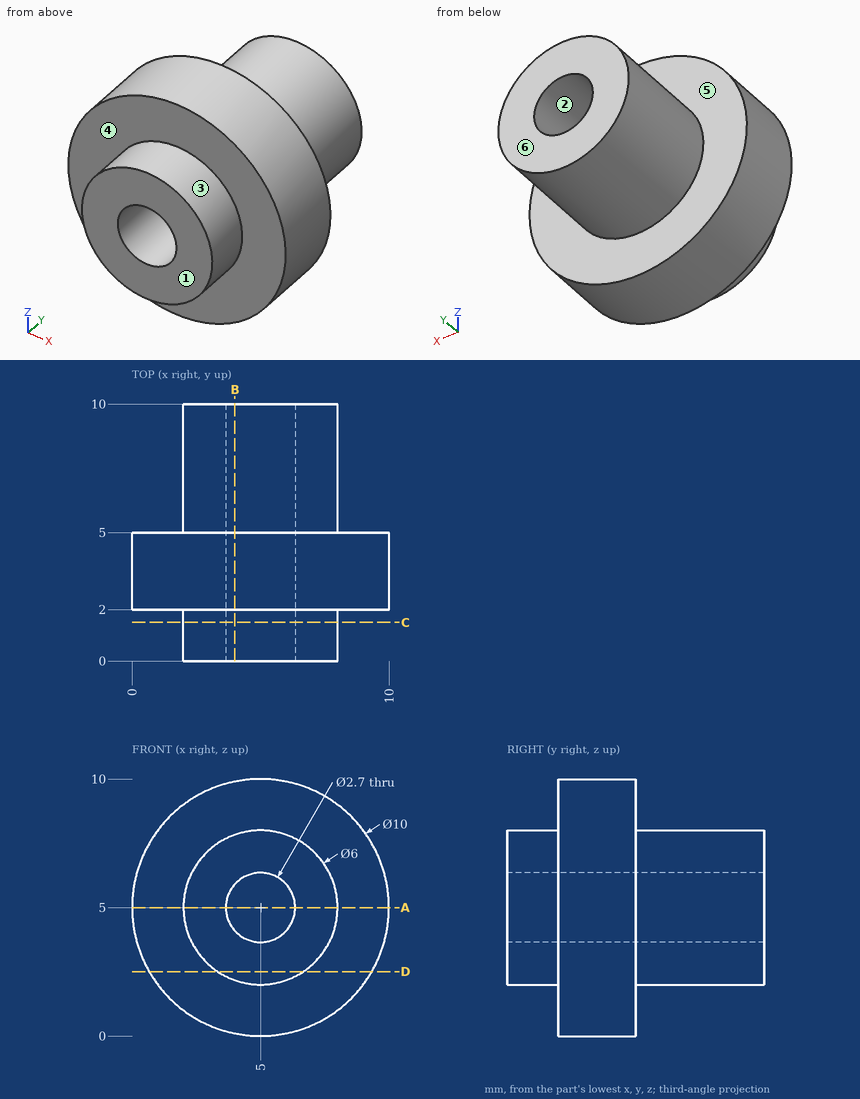
Check sheet for the drawn part. Datum: minimum x, y, z corner. Units: mm. A direction names the side the tool comes from. Round coordinates to 2 decimals unless told otherwise and drop trailing zeros. Write each loop counter-clockwise with the first axis right and the second up, starting at its lowest first coordinate (ties: lowest second). Pieces come first, ordered by that corner, then holes. Notation, with made-up numbers: (66, 14.25) -> (110, 14.25) arc R12 ccw to (110, 20.25) -> close; hole circle Ø6 at (17, 66). An arc over 180 degrees is marked (long way). Write each question's results on one line, items separated by ' | '.
Q1. Access from +Z, -Z, +X, -X, +Y, -Y to the whole of each face (thin tool, end or side, straight path). Record for the marked faces 4, 5 and 6.
Derived:
face 4: -Y | face 5: +Y | face 6: +Z, -Z, +X, -X, +Y
Q2. Sectioned sample at B-B, the plane x = 4. Record the boundary of the cut face in (y, z).
Derived:
outline: (0, 2.17) -> (2, 2.17) -> (2, 0.1) -> (5, 0.1) -> (5, 2.17) -> (10, 2.17) -> (10, 4.09) -> (0, 4.09) -> close; (0, 5.91) -> (10, 5.91) -> (10, 7.83) -> (5, 7.83) -> (5, 9.9) -> (2, 9.9) -> (2, 7.83) -> (0, 7.83) -> close
Q3. Sectioned sample at D-D, the plane z = 2.5. Record the boundary of the cut face in (x, y).
Derived:
outline: (0.67, 2) -> (3.34, 2) -> (3.34, 0) -> (6.66, 0) -> (6.66, 2) -> (9.33, 2) -> (9.33, 5) -> (6.66, 5) -> (6.66, 10) -> (3.34, 10) -> (3.34, 5) -> (0.67, 5) -> close
Q4. Draft check along X on the marked faces 1, 2 and 3. Enter one of: released by +X, released by -X, zero draft, split by the parting line, or undercut.
Derived:
face 1: zero draft | face 2: undercut | face 3: split by the parting line
Q5. Sectioned sample at C-C, the plane y = 1.5. Record the boundary of the cut face in (x, z), and give its area (3 significant figures).
Derived:
outline: circle Ø6 at (5, 5); hole circle Ø2.7 at (5, 5) | area: 22.5 mm²
Q6. Go/stop test with flat-tipped pins: pin 1 Ø1 at (x, y) = (2.5, 4.5) entering from -Z; pin 2 Ø1.5 at (x, z) = (5.5, 9) entering from +Y; pin 3 Ø1.5 at (x, y) = (8.5, 4.5) entering from +Z; pin 4 Ø2 at (x, z) = (5, 5) entering from -Y. Record where each tip stops, or that it passes through.
Derived:
pin 1: stops at z = 0.42 | pin 2: stops at y = 5 | pin 3: stops at z = 9.18 | pin 4: passes through
Q7. Sectioned sample at A-A, the plane z = 5. Record the boundary of the cut face in (x, y).
Derived:
outline: (0, 2) -> (2, 2) -> (2, 0) -> (3.65, 0) -> (3.65, 10) -> (2, 10) -> (2, 5) -> (0, 5) -> close; (6.35, 0) -> (8, 0) -> (8, 2) -> (10, 2) -> (10, 5) -> (8, 5) -> (8, 10) -> (6.35, 10) -> close
Q8. Thickness scan on probe 1 along X at (y, z) = (3, 5); probe 2 along Z at (x, y) = (5, 7.5). Record the ranges inside material, lowest first.
Derived:
probe 1: x = 0 to 3.65, 6.35 to 10 | probe 2: z = 2 to 3.65, 6.35 to 8
